```python
from build123d import *

# Parameters (mm, degrees)
BOSS_EXTRUDE1_DEPTH = 40
SHELL1_T            = -2.5
SKETCH2_R           = 5
CUT_EXTRUDE1_DEPTH  = 40
SKETCH3_R           = 2.5
CUT_EXTRUDE2_DEPTH  = 2.5
SKETCH4_W           = 6
SKETCH4_H           = 3
CUT_EXTRUDE3_DEPTH  = 40
CIRPATTERN1_COUNT   = 6


with BuildPart() as part:
    # Sketch1 → Boss-Extrude1 (new body)
    with BuildSketch(Plane(origin=(0, 0, 0), x_dir=(1, 0, 0), z_dir=(0, 1, 0))):
        Polygon((34.641016151, 20), (0, 40), (-34.641016151, 20), (-34.641016151, -20), (0, -40), (34.641016151, -20), align=None)
    extrude(amount=BOSS_EXTRUDE1_DEPTH)

    # Shell1
    shell1_openings = [part.faces().sort_by_distance(p)[0] for p in [
        (0, 40, 0),
    ]]
    offset(amount=SHELL1_T, openings=shell1_openings, kind=Kind.INTERSECTION)

    # Sketch2 → Cut-Extrude1 (cut)
    with BuildSketch(Plane.XZ):
        with Locations(Location((0, 0, 0), (0, 0, 270))):
            Circle(SKETCH2_R)
    extrude(amount=-CUT_EXTRUDE1_DEPTH, mode=Mode.SUBTRACT)

    # Sketch3 → Cut-Extrude2 (cut)
    with BuildSketch(Plane.ZY.offset(34.641016151)):
        with Locations((-15.137351835, 34.838276852)):
            Circle(SKETCH3_R)
        with Locations((14.232401454, 34.838276852)):
            Circle(SKETCH3_R)
    cut_extrude2 = extrude(amount=-CUT_EXTRUDE2_DEPTH, mode=Mode.SUBTRACT)

    # Sketch4 → Cut-Extrude3 (cut)
    with BuildSketch(Plane.ZY.offset(34.641016151)):
        with Locations((0, 20)):
            Rectangle(SKETCH4_W, SKETCH4_H)
    cut_extrude3 = extrude(amount=-CUT_EXTRUDE3_DEPTH, mode=Mode.SUBTRACT)

    # CirPattern1: Cut-Extrude2, Cut-Extrude3 ×6 about axis
    cirpattern1_axis = Axis((0, 0, 0), (0, 1, 0))
    add([cut_extrude2.rotate(cirpattern1_axis, i * 360 / CIRPATTERN1_COUNT) for i in range(1, CIRPATTERN1_COUNT)], mode=Mode.SUBTRACT)
    add([cut_extrude3.rotate(cirpattern1_axis, i * 360 / CIRPATTERN1_COUNT) for i in range(1, CIRPATTERN1_COUNT)], mode=Mode.SUBTRACT)


solid = part.part
```
Could you check a few things on this model? Use its own coordinates, in mm. A direction names the side the tool comes from. Coordinates: 2 decimals unless noted, no trailing zeros. Loops run counter-clockwise (first coordinate to the right, second up) from the corner with the lowest first, then second, coordinate; pieces in that order, holes last. Notation, with made-up numbers: M 31.5,45 L 47.5,45 A18 ccw 47.5,60 Z; hole C -25.75,-16.5 d2. An arc over 180 degrees is marked long. Put each result on its own line as item: value. Start each with the question number.
(1) Suppose I cut it at A-A on z = 0. Please give me the cut outline in (x, y).
(2) For faces 4 (the face through (-16.295, 16.821, 27.705)), 5 (the face through (-19.3, 19.98, 27.43)), 6 (the face through (-14.106, 19.979, -30.433)), 7 (the face through (17, 18.5, 29)), which set-ups out of +Z, -Z, +X, -X, +Y, -Y let a thin tool reach every point of the face, with its end or its side?
(3) Suppose I cut it at B-B on y = 11.5. Please give me the cut outline in (x, z).
(4) Thinking about a two-plate mould opening in X: for faces 1 (the face through (14.106, 19.979, -30.433)), 2 (the face through (33.409, 36.946, 13.793)), 3 (the face through (32.141, 17, 0)), which applies, pulls with the +X half, pulls with the -X half, needs draft (parallel to the pull), parting line crosses it, or undercut?
(5) Suppose I cut it at D-D on x = -9.5. Please give me the cut outline in (y, z).
(6) I need wall thicknesses on line 1 (X direction, y = 1, z = 0); line 2 (X direction, y = 36.5, z = 2.5); line 3 (Y direction, x = -0.5, z = -28.5). Which ranges of each line are inside material? Lowest first, please. Write a range as from..to.
(7) Suppose I cut it at C-C on x = -17.5. Please give me the cut outline in (y, z).
(8) Will these pins go through, and if not, where does the flat tip stop? P1, Ø0.8, axis at x = 34, y = 20.5, coming from the +Z side; P2, Ø3, axis at x = 34, y = 19.5, coming from the -Z side; P3, Ø4, axis at x = 4, z = -30, coming from the +Y side.
Solutions:
1. outline: M -34.64,0 L -5,0 L -5,2.5 L -32.14,2.5 L -32.14,18.5 L -34.64,18.5 Z; M -34.64,21.5 L -32.14,21.5 L -32.14,40 L -34.64,40 Z; M 5,0 L 34.64,0 L 34.64,18.5 L 32.14,18.5 L 32.14,2.5 L 5,2.5 Z; M 32.14,21.5 L 34.64,21.5 L 34.64,40 L 32.14,40 Z
2. face 4: +Y
2. face 5: +Z
2. face 6: -X
2. face 7: none
3. outline: M -34.64,-20 L 0,-40 L 34.64,-20 L 34.64,20 L 0,40 L -34.64,20 Z; hole M -32.14,-18.56 L 0,-37.11 L 32.14,-18.56 L 32.14,18.56 L 0,37.11 L -32.14,18.56 Z
4. face 1: pulls with the +X half
4. face 2: needs draft
4. face 3: undercut
5. outline: M 0,-34.52 L 40,-34.52 L 40,-31.63 L 2.5,-31.63 L 2.5,31.63 L 40,31.63 L 40,34.52 L 0,34.52 Z
6. line 1: x = -34.64..-5, 5..34.64
6. line 2: x = -34.64..-32.14, 32.14..34.64
6. line 3: y = 0..2.5
7. outline: M 0,-29.9 L 18.5,-29.9 L 18.5,-27.01 L 2.5,-27.01 L 2.5,27.01 L 18.5,27.01 L 18.5,29.9 L 0,29.9 Z; M 21.5,-29.9 L 40,-29.9 L 40,-27.01 L 21.5,-27.01 Z; M 21.5,27.01 L 40,27.01 L 40,29.9 L 21.5,29.9 Z
8. P1: stops at z = 20.6
8. P2: stops at z = -21.24
8. P3: stops at y = 2.5
